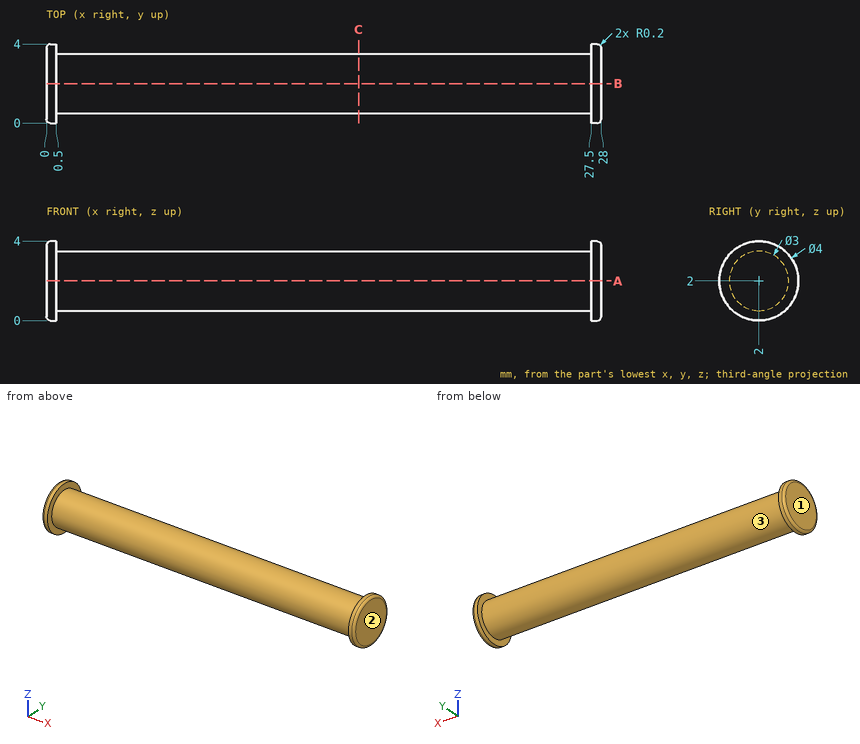
Can you work these out from the drawing? Everything is in mm from the part's minimum corner. Give positions to 0.01 mm unless a question says otherwise; leave off trailing zeros. Loops run counter-clockwise (first coordinate to the right, second up) from the corner with the lowest first, then second, coordinate; pieces in that order, holes last. Notation, with made-up numbers: (9, 50.25) -> (34, 50.25) arc R19 cw to (34, 56.25) -> close; hole circle Ø4 at (-29.75, 45). An arc over 180 degrees is marked (long way). Return JSON: item names as keys, results as strings.
Item 1: If we section it at A-A on z = 2: List the corners of the cut face in (x, y) for me, plus the area to 3 significant figures.
Geometry results:
{"outline": "(0, 0.2) arc R0.2 ccw to (0.2, 0) -> (0.5, 0) -> (0.5, 0.5) -> (27.5, 0.5) -> (27.5, 0) -> (27.8, 0) arc R0.2 ccw to (28, 0.2) -> (28, 3.8) arc R0.2 ccw to (27.8, 4) -> (27.5, 4) -> (27.5, 3.5) -> (0.5, 3.5) -> (0.5, 4) -> (0.2, 4) arc R0.2 ccw to (0, 3.8) -> close", "area": "85.0 mm²"}
Item 2: We'd pull the mould along X, two halves only. Please class the marked faces 1, 2 and 3: +X half, -X half, draft (parallel to the pull), parting line (faces both ways), or undercut.
Geometry results:
{"face 1": "-X half", "face 2": "+X half", "face 3": "undercut"}
Item 3: I need wall thicknesses on L1, parallel to X at y = 3.3, z = 0.75; L2, parallel to Z at x = 27.25, y = 2.05; L3, parallel to Z at x = 19.25, y = 1.15. Which ranges of each line are inside material? Lowest first, please. Write a range as from..to.
Geometry results:
{"L1": "x = 0..0.5, 27.5..28", "L2": "z = 0.5..3.5", "L3": "z = 0.76..3.24"}
Item 4: If we section it at C-C on x = 15.75: List the corners of the cut face in (y, z) for me.
Geometry results:
{"outline": "circle Ø3 at (2, 2)"}
Item 5: I'm going to push flat-ended pins straight in: pin 1 (2 mm diameter, centred on x = 23, y = 1, fed in from +Z); pin 2 (1.5 mm diameter, centred on x = 21.5, z = 2, fed in from +Y). Where does each tip first touch, or does it pass through?
Geometry results:
{"pin 1": "stops at z = 3.5", "pin 2": "stops at y = 3.5"}
